Part print with two shaded views. Sizes in mm from the minimum x, y, z corner. Round coordinates to 2 decimals unless told otherwise and drop trailing zeros. Order: outer loops, then holes, each group sorted by start corner. A loop starts at its lowest first (then second) coordinate and runs counter-clockwise, first axis right, second up. Notation, with made-up numbers: M 27,73.5 L 48,73.5 A29 cw 48,98.5 Z; hole C -11,47 d6. An arc over 180 degrees is marked long. Answer as a JSON object with one key per item and string values.
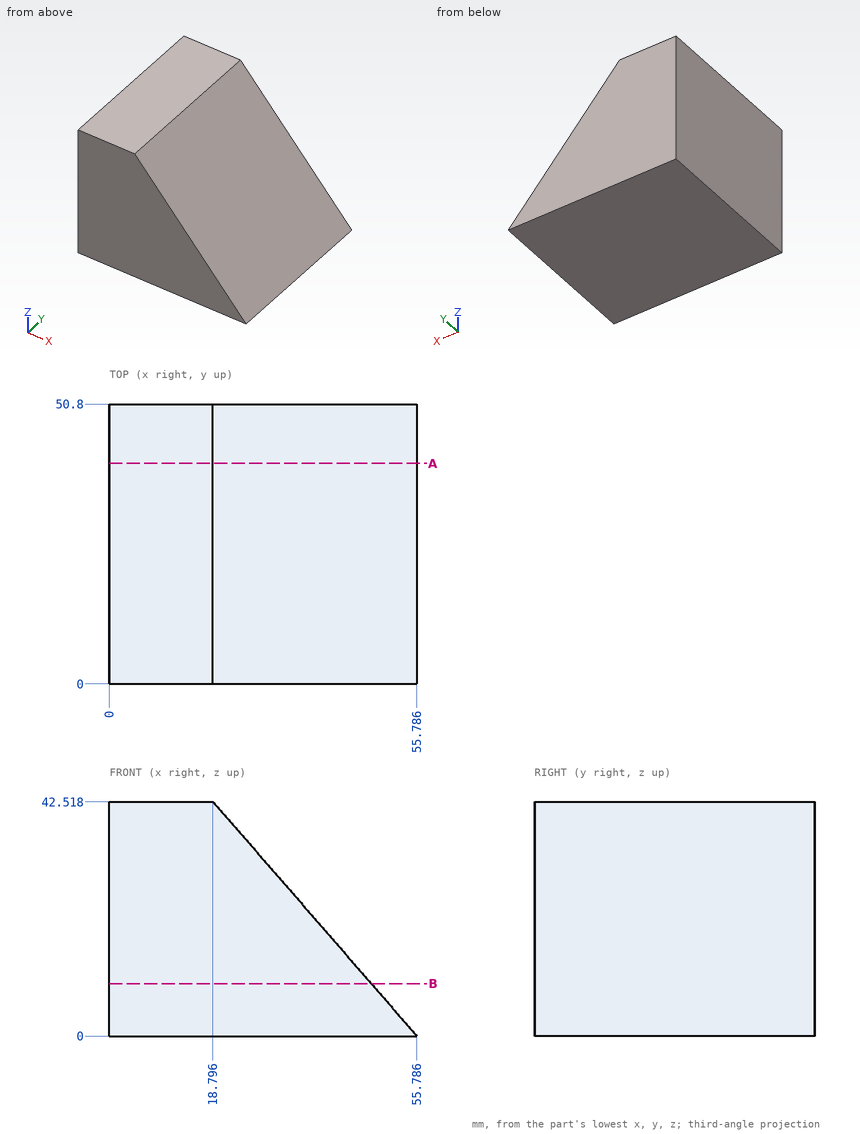
Item 1: Saw through at A-A on y = 40. List the corners of the cut face in (x, z).
Worked answers:
{"outline": "M 0,0 L 55.79,0 L 18.8,42.52 L 0,42.52 Z"}
Item 2: Drop flat-ended pins along their axis: pin 1 Ø6 at (y, z) = (10, 37.5) entering from +X; pin 2 Ø12 at (x, y) = (32, 11.5) entering from +Z; pin 3 Ø6 at (x, y) = (23.5, 23.5) entering from +Z. Give the stop position or say it passes through.
Worked answers:
{"pin 1": "stops at x = 25.77", "pin 2": "stops at z = 34.24", "pin 3": "stops at z = 40.56"}
Item 3: Wall check: line 1 along X through (y, z) = (32.5, 34) (1 decimal); line 2 along X through (y, z) = (48.5, 29) (1 decimal); line 3 along Z through (x, y) = (32.5, 27.5) (1 decimal). Give the ranges that are in metal, low to high. Write a range as [from, to].
Worked answers:
{"line 1": "x = [0, 26.2]", "line 2": "x = [0, 30.6]", "line 3": "z = [0, 26.8]"}
Item 4: Saw through at B-B on z = 9.5. List the corners of the cut face in (x, y).
Worked answers:
{"outline": "M 0,0 L 47.52,0 L 47.52,50.8 L 0,50.8 Z"}
